Input: dimensioned drawing with shaded views. Units: mm. Origin: part minimum x, y, z. Coordinates: 2 decimals unless noted, no trailing zeros. Write each loop counter-clockwise with the first axis right and the second up, starting at its lowest first coordinate (ties: lowest second). Pieces come first, ordered by that corner, then holes. Notation, with made-up numbers: M 41.5,-24 L 50.5,-24 A20 cw 50.5,-8 Z; hole C 82.25,80 d9. An arc over 180 degrees is marked long. Write each question's results on one line, items separated by ' | '. Start each with the question number.
1. Ray query, probe 1 along Z at (x, y) = (257.5, 5.5) (1 decimal). Return the intervals inside material, ascending.
2. Section query B-B, the plane x = 304. Output: boundary loops of the cut face in (y, z) (1 decimal).
3. First-contact query: pin 1 (2.5 mm diameter, centred on x = 174, y = 4.5, fed in from -Z); pin 2 (2.5 mm diameter, centred on y = 4, z = 417, fed in from +X); pin 3 (4 mm diameter, centred on y = 4.5, z = 430, fed in from -X). Flat tips, straight axial feed; report the tip coordinate or a pass-through.
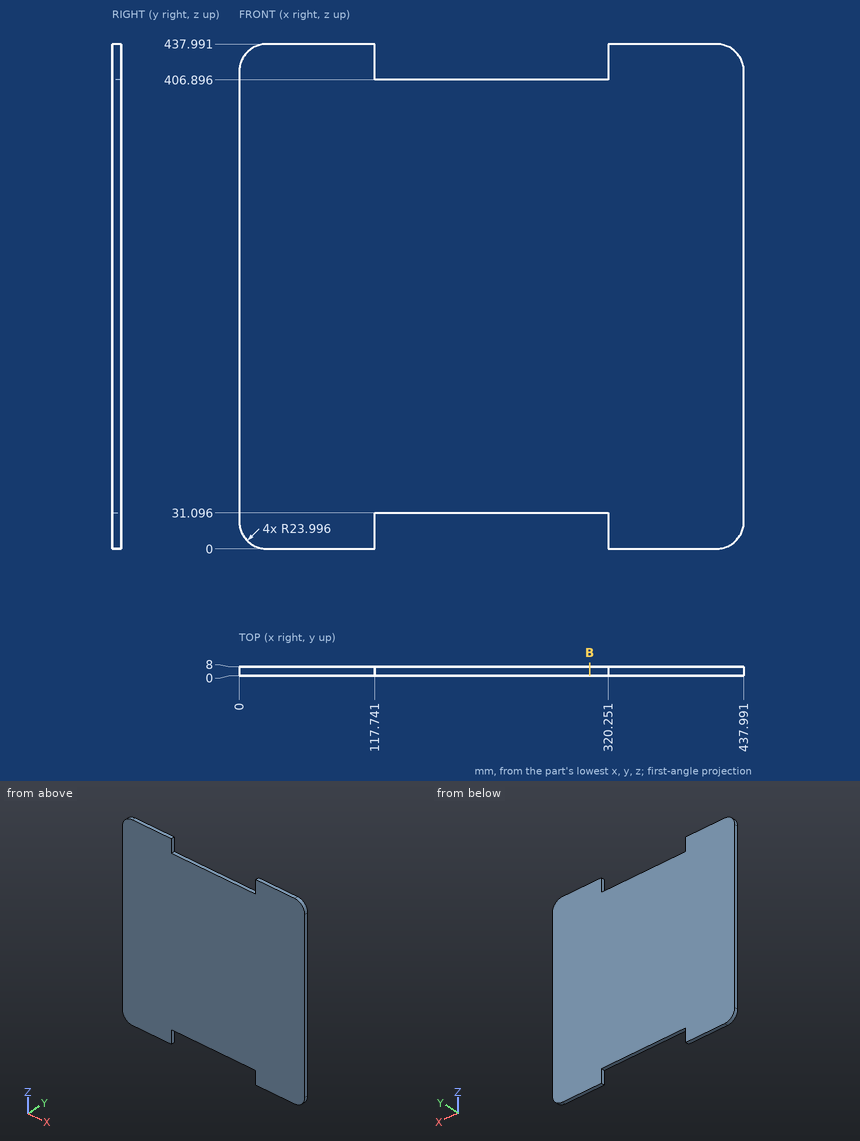
Answer:
1) probe 1: 31.1 to 406.9
2) outline: M 0,31.1 L 8,31.1 L 8,406.9 L 0,406.9 Z
3) pin 1: z = 31.1 | pin 2: x = 437.93 | pin 3: x = 4.51
